Source: CAD feature listing. Evaluate the final solid. Frame: model axes, mm. A direction names the side the tool comes from. Round coordinates to 2 decimals unless told otherwise and drop trailing zeros. Order: outer loops, then holes, each group sorted by start corner. A loop starts at its lowest first (then second) coordinate and runs counter-clockwise, first axis right, second up. Notation, with made-up numbers: M 47.25,44 L 74.25,44 A31 cw 74.25,79 Z; hole C 78.5,27.25 d5. An arc over 180 degrees is marked long. Use one line per item in the form item = value. Start each with the question number.
Q1. Contact query for flat-ended pins moving along their axis: pin 1 (0.8 mm diameter, centred on x = 8, y = 1.5, fed in from +Z); pin 2 (0.8 mm diameter, centred on x = 8.5, y = 1.5, fed in from -Z); pin 3 (1.8 mm diameter, centred on x = 0.5, z = -1, fed in from +Y). Output: stop coordinate, or through.
Q2. Section B-B (y = 1.3). Return the cut outline in (x, z).
Q3. Section A-A (x = 0). Return the cut outline in (y, z).
Q4. Section C-C (x = 5.75). Return the cut outline in (y, z), plus the area to 3 significant figures.
Q5. Section D-D (y = 3.9). Return the cut outline in (x, z), plus the area to 3 significant figures.
Q6. Reachability of faces 1 (the flat face through (2.3, 5, 0.2)), 2 (the cylindrical face through (-1.806, 3.356, -0.401)), 3 (the flat face through (9, 1, 1)) from +Z, -Z, +X, -X, +Y, -Y: full face, straight path, thin tool, end or side. Return the list, or none.
Q7. Material intervals for probe 1 along X at (y, z) = (1.15, 0); probe 2 along X at (y, z) = (3.8, 0); probe 3 along Z at (x, y) = (6, 1.1), sorted ascending.
Q8. Pull-direction query (X, two-part tool) for faces 4 (the cylindrical face through (3.5, 1.3, 0)), 5 (the flat face through (6, 0, 2)), 6 (the cylindrical face through (15.304, 1.268, 1.883)); classes: pulls with the +X half, pulls with the -X half, needs draft (parallel to the pull), parting line crosses it, or undercut.
from build123d import *

# Parameters (mm, degrees)
SKETCH1_R           = 1.25
BOSS_EXTRUDE1_DEPTH = 2.5
SKETCH2_R           = 3.5
SKETCH2_R_2         = 1.25
BOSS_EXTRUDE2_DEPTH = 2.5
CUT_EXTRUDE1_START  = -3
SKETCH3_R           = 1.85
SKETCH3_R_2         = 1.25
CUT_EXTRUDE1_DEPTH  = 3
CHAMFER1_SIZE       = 0.25
CUT_EXTRUDE2_DEPTH  = 3
FILLET1_R           = 2.5


with BuildPart() as part:
    # Sketch1 → Boss-Extrude1 (new body)
    with BuildSketch(Plane(origin=(0, 0, 0), x_dir=(1, 0, 0), z_dir=(0, 1, 0))):
        with BuildLine():
            ThreePointArc((0.219829752, 3.49308959), (-3.5, 0), (0.219829752, -3.49308959))
            Line((0.219829752, -3.49308959), (16, -2.5))
            Line((16, -2.5), (16, 2.5))
            Line((16, 2.5), (0.219829752, 3.49308959))
        make_face()
        with Locations(Location((0, 0, 0), (0, 0, 270))):
            Circle(SKETCH1_R, mode=Mode.SUBTRACT)
    extrude(amount=BOSS_EXTRUDE1_DEPTH)

    # Sketch2 → Boss-Extrude2 (add)
    with BuildSketch(Plane(origin=(0, 2.5, 0), x_dir=(1, 0, 0), z_dir=(0, 1, 0))):
        with Locations(Location((0, 0, 0), (0, 0, 86.398967731))):
            Circle(SKETCH2_R)
        with Locations(Location((0, 0, 0), (0, 0, 270))):
            Circle(SKETCH2_R_2, mode=Mode.SUBTRACT)
    extrude(amount=BOSS_EXTRUDE2_DEPTH)

    # Sketch3 → Cut-Extrude1 (cut)
    with BuildSketch(Plane(origin=(0, 5, 0), x_dir=(1, 0, 0), z_dir=(0, 1, 0)).offset(CUT_EXTRUDE1_START)):
        with Locations(Location((0, 0, 0), (0, 0, 270))):
            Circle(SKETCH3_R)
        with Locations(Location((0, 0, 0), (0, 0, 270))):
            Circle(SKETCH3_R_2, mode=Mode.SUBTRACT)
    extrude(amount=CUT_EXTRUDE1_DEPTH, mode=Mode.SUBTRACT)

    # Chamfer1
    chamfer1_edges = [part.edges().sort_by_distance(p)[0] for p in [
        (0, 5, -1.85),
    ]]
    chamfer(chamfer1_edges, length=CHAMFER1_SIZE)

    # Sketch4 → Cut-Extrude2 (cut)
    with BuildSketch(Plane(origin=(0, 2.5, 0), x_dir=(1, 0, 0), z_dir=(0, 1, 0))):
        with BuildLine():
            Line((4.5, 1), (12.5, 1))
            ThreePointArc((12.5, 1), (13.5, 0), (12.5, -1))
            Line((12.5, -1), (4.5, -1))
            ThreePointArc((4.5, -1), (3.5, 0), (4.5, 1))
        make_face()
    extrude(amount=-CUT_EXTRUDE2_DEPTH, mode=Mode.SUBTRACT)

    # Fillet1
    fillet1_edges = [part.edges().sort_by_distance(p)[0] for p in [
        (16, 1.25, -2.5),
        (16, 1.25, 2.5),
    ]]
    fillet(fillet1_edges, radius=FILLET1_R)


solid = part.part
Results list:
q1.pin_1 = 3.03
q1.pin_2 = -3
q1.pin_3 = 4.92
q2.outline = M 0.22,-3.49 L 13.66,-2.65 A2.5 ccw 16,-0.15 L 16,0.15 A2.5 ccw 13.66,2.65 L 0.22,3.49 A3.5 ccw long Z; hole C 0,0 d2.5; hole M 4.5,-1 L 12.5,-1 A1 ccw 12.5,1 L 4.5,1 A1 ccw Z
q3.outline = M 0,-3.5 L 5,-3.5 L 5,-2.1 L 4.75,-1.85 L 2,-1.85 L 2,-1.25 L 0,-1.25 Z; M 0,1.25 L 2,1.25 L 2,1.85 L 4.75,1.85 L 5,2.1 L 5,3.5 L 0,3.5 Z
q4.outline = M 0,-3.15 L 2.5,-3.15 L 2.5,-1 L 0,-1 Z; M 0,1 L 2.5,1 L 2.5,3.15 L 0,3.15 Z
q4.area = 10.7 mm2
q5.outline = C 0,0 d7; hole C 0,0 d3.7
q5.area = 27.7 mm2
q6.face_1 = +Z, -Z, +X, -X, +Y
q6.face_2 = +Y
q6.face_3 = +Y, -Y
q7.probe_1 = -3.5 to -1.25, 1.25 to 3.5, 13.5 to 16
q7.probe_2 = -3.5 to -1.85, 1.85 to 3.5
q7.probe_3 = -3.13 to -1, 1 to 3.13
q8.face_4 = undercut
q8.face_5 = needs draft
q8.face_6 = pulls with the +X half
